```python
from build123d import *

# Parameters (mm, degrees)
SKETCH1_R          = 8
EXTRUDE1_DEPTH     = 40
SKETCH2_W          = 5
SKETCH2_H          = 3.872152866
CUT_EXTRUDE1_DEPTH = 25
FILLET1_R          = 2.5
CHAMFER1_SIZE      = 1
SKETCH3_R          = 10
EXTRUDE2_DEPTH     = 15
CHAMFER2_SIZE      = 2
SKETCH4_R          = 12.3
EXTRUDE3_DEPTH     = 12
CHAMFER3_SIZE      = 2
SKETCH5_R          = 12.5
EXTRUDE4_DEPTH     = 13
SKETCH6_R          = 14.5
EXTRUDE5_DEPTH     = 20
SKETCH10_W         = 5
SKETCH10_H         = 6.103543743
CUT_EXTRUDE2_DEPTH = 14.4
FILLET2_R          = 2.5
SKETCH9_R          = 8
EXTRUDE6_DEPTH     = 54
SKETCH11_W         = 4
SKETCH11_H         = 18
CUT_EXTRUDE3_DEPTH = 156.968746869
FILLET3_R          = 2
SKETCH12_R         = 7.975
EXTRUDE7_DEPTH     = 23
CHAMFER4_SIZE      = 1


# Some blends are built 0.0001 mm under size
with BuildPart() as part:
    # Sketch1 → Extrude1 (new body)
    with BuildSketch(Plane.XY):
        Circle(SKETCH1_R)
    extrude(amount=-EXTRUDE1_DEPTH)

    # Sketch2 → Cut-Extrude1 (cut)
    with BuildSketch(Plane.XY):
        with Locations((0, 6.936076433)):
            Rectangle(SKETCH2_W, SKETCH2_H)
    extrude(amount=-CUT_EXTRUDE1_DEPTH, mode=Mode.SUBTRACT)

    # Fillet1
    fillet1_edges = [part.edges().sort_by_distance(p)[0] for p in [
        (2.5, 6.299671038, -25),
        (-2.5, 6.299671038, -25),
    ]]
    fillet(fillet1_edges, radius=FILLET1_R - 0.0001)  # a hair under: the kernel refuses the full size

    # Chamfer1
    chamfer1_edges = [part.edges().sort_by_distance(p)[0] for p in [
        (-4.69041576, -6.480740698, 0),
    ]]
    chamfer(chamfer1_edges, length=CHAMFER1_SIZE)

    # Sketch3 → Extrude2 (add)
    with BuildSketch(Plane(origin=(0, 0, -40), x_dir=(-1, 0, 0), z_dir=(0, 0, -1))):
        Circle(SKETCH3_R)
    extrude(amount=EXTRUDE2_DEPTH)

    # Chamfer2
    chamfer2_edges = [part.edges().sort_by_distance(p)[0] for p in [
        (10, 0, -40),
    ]]
    chamfer(chamfer2_edges, length=CHAMFER2_SIZE - 0.0001)  # a hair under: the kernel refuses the full size

    # Sketch4 → Extrude3 (add)
    with BuildSketch(Plane(origin=(0, 0, -55), x_dir=(-1, 0, 0), z_dir=(0, 0, -1))):
        Circle(SKETCH4_R)
    extrude(amount=EXTRUDE3_DEPTH)

    # Chamfer3
    chamfer3_edges = [part.edges().sort_by_distance(p)[0] for p in [
        (12.3, 0, -55),
    ]]
    chamfer(chamfer3_edges, length=CHAMFER3_SIZE)

    # Sketch5 → Extrude4 (add)
    with BuildSketch(Plane(origin=(0, 0, -67), x_dir=(-1, 0, 0), z_dir=(0, 0, -1))):
        with Locations(Location((0, 0, 0), (0, 0, 180))):
            Circle(SKETCH5_R)
    extrude(amount=EXTRUDE4_DEPTH)

    # Sketch6 → Extrude5 (add)
    with BuildSketch(Plane(origin=(0, 0, -80), x_dir=(-1, 0, 0), z_dir=(0, 0, -1))):
        Circle(SKETCH6_R)
    extrude(amount=EXTRUDE5_DEPTH)

    # Sketch10 → Cut-Extrude2 (cut)
    with BuildSketch(Plane.XY.offset(-55)):
        with Locations((0, 13.551771871)):
            Rectangle(SKETCH10_W, SKETCH10_H)
    extrude(amount=-CUT_EXTRUDE2_DEPTH, mode=Mode.SUBTRACT)

    # Fillet2
    # the kernel refuses this fillet: 2.5 mm, written as the material it adds along each edge
    with BuildSketch(Plane(origin=(2.5, 18.497448714, -69.4), x_dir=(0, 0, 1), z_dir=(0, -1, 0))) as fillet2_piece_1_section:
        with BuildLine():
            CenterArc((FILLET2_R, FILLET2_R), FILLET2_R, 180, 90)
            Line((0, FILLET2_R), (0, 0))
            Line((0, 0), (FILLET2_R, 0))
        make_face()
    fillet2_piece_1 = extrude(amount=14.247448714, mode=Mode.PRIVATE)
    fillet2_piece_1 = fillet2_piece_1 & Plane(origin=(0, 0, -68.840122938), x_dir=(1, 0, 0), z_dir=(0, 0, 1)) * Cylinder(12.5, 39, mode=Mode.PRIVATE)
    fillet2_piece_1 = split(fillet2_piece_1, bisect_by=Plane(origin=(1.944027658, 12.237538555, -67), z_dir=(0, 0, -1)), keep=Keep.TOP, mode=Mode.PRIVATE)
    add(fillet2_piece_1)
    with BuildSketch(Plane(origin=(2.5, 18.497448714, -69.4), x_dir=(0, 0, 1), z_dir=(0, -1, 0))) as fillet2_piece_2_section:
        with BuildLine():
            CenterArc((FILLET2_R, FILLET2_R), FILLET2_R, 180, 90)
            Line((0, FILLET2_R), (0, 0))
            Line((0, 0), (FILLET2_R, 0))
        make_face()
    fillet2_piece_2 = extrude(amount=14.247448714, mode=Mode.PRIVATE)
    fillet2_piece_2 = fillet2_piece_2 & Plane(origin=(0, 0, -66.975002686), x_dir=(-1, 0, 0), z_dir=(0, 0, 1)) * Cylinder(12.3, 39, mode=Mode.PRIVATE)
    add(fillet2_piece_2)
    with BuildSketch(Plane(origin=(-2.5, 4.25, -69.4), x_dir=(1, 0, 0), z_dir=(0, 1, 0))) as fillet2_piece_3_section:
        with BuildLine():
            CenterArc((FILLET2_R, -FILLET2_R), FILLET2_R, 90, 90)
            Line((0, -FILLET2_R), (0, 0))
            Line((0, 0), (FILLET2_R, 0))
        make_face()
    fillet2_piece_3 = extrude(amount=14.247448714, mode=Mode.PRIVATE)
    fillet2_piece_3 = fillet2_piece_3 & Plane(origin=(0, 0, -68.853362748), x_dir=(1, 0, 0), z_dir=(0, 0, 1)) * Cylinder(12.5, 39, mode=Mode.PRIVATE)
    fillet2_piece_3 = split(fillet2_piece_3, bisect_by=Plane(origin=(-1.922744222, 11.319637846, -67), z_dir=(0, 0, -1)), keep=Keep.TOP, mode=Mode.PRIVATE)
    add(fillet2_piece_3)
    with BuildSketch(Plane(origin=(-2.5, 4.25, -69.4), x_dir=(1, 0, 0), z_dir=(0, 1, 0))) as fillet2_piece_4_section:
        with BuildLine():
            CenterArc((FILLET2_R, -FILLET2_R), FILLET2_R, 90, 90)
            Line((0, -FILLET2_R), (0, 0))
            Line((0, 0), (FILLET2_R, 0))
        make_face()
    fillet2_piece_4 = extrude(amount=14.247448714, mode=Mode.PRIVATE)
    fillet2_piece_4 = fillet2_piece_4 & Plane(origin=(0, 0, -66.975002689), x_dir=(-1, 0, 0), z_dir=(0, 0, 1)) * Cylinder(12.3, 39, mode=Mode.PRIVATE)
    add(fillet2_piece_4)

    # Sketch9 → Extrude6 (add)
    with BuildSketch(Plane(origin=(0, 0, -100), x_dir=(-1, 0, 0), z_dir=(0, 0, -1))):
        with Locations(Location((0, 0, 0), (0, 0, 108.209956864))):
            Circle(SKETCH9_R)
    extrude(amount=EXTRUDE6_DEPTH)

    # Sketch11 → Cut-Extrude3 (cut, through all)
    with BuildSketch(Plane(origin=(0, -5.5, 0), x_dir=(-1, 0, 0), z_dir=(0, 1, 0))):
        with Locations((0, -110)):
            Rectangle(SKETCH11_W, SKETCH11_H)
    extrude(amount=-CUT_EXTRUDE3_DEPTH, mode=Mode.SUBTRACT)

    # Fillet3
    fillet3_edges = [part.edges().sort_by_distance(p)[0] for p in [
        (-2, -6.622983346, -119),
        (2, -6.622983346, -119),
        (-2, -6.622983346, -101),
        (2, -6.622983346, -101),
    ]]
    fillet(fillet3_edges, radius=FILLET3_R - 0.0001)  # a hair under: the kernel refuses the full size

    # Sketch12 → Extrude7 (add)
    with BuildSketch(Plane(origin=(0, 0, -154), x_dir=(-1, 0, 0), z_dir=(0, 0, -1))):
        Circle(SKETCH12_R)
    extrude(amount=EXTRUDE7_DEPTH)

    # Chamfer4
    chamfer4_edges = [part.edges().sort_by_distance(p)[0] for p in [
        (7.975, 0, -177),
    ]]
    chamfer(chamfer4_edges, length=CHAMFER4_SIZE)


solid = part.part
```
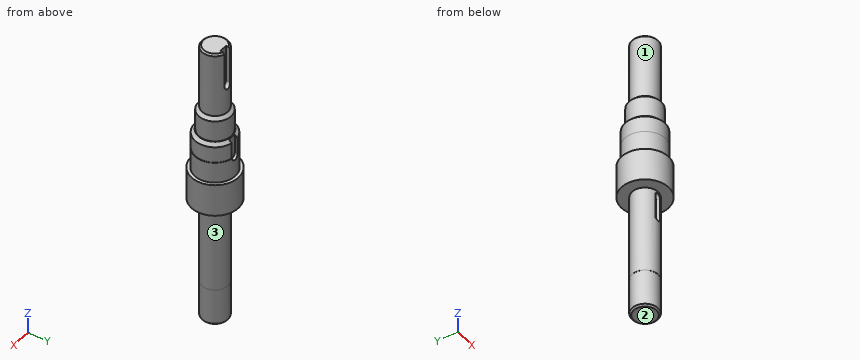
CAD build for the part. Positions are in the model's coordinates, mm. Face numbers are marked on the shaded views. A direction names the side the tool comes from. Coordinates: 2 decimals unless noted, no trailing zeros. Write each loop counter-clockwise with the first axis right and the second up, starting at its lowest first coordinate (ties: lowest second). Pieces come first, ordered by that corner, then holes.
(1) Flat gauge pins, fed straight in: pin 1 (1.8 mm diameter, centred on y = -7, z = -109.5, fed in from -X); pin 2 (2 mm diameter, centred on x = -6.5, z = -93.5, fed in from -Y); pin 3 (10 mm diameter, centred on x = 7, y = 0.5, fed in from -Z); pin 4 (2.5 mm diameter, centred on y = -7, z = -111.5, fed in from +X). Where does each tip first touch, or does it go through?
(2) Cut at C-C, the plane z = -50. List the corners of the cut face in (x, y).
(3) Cut at A-A, the plane z = -83.5. List the corners of the cut face in (x, y), and give its area (3 significant figures).
(4) Cut at B-B, the plane z = -108. List the corners of the cut face in (x, y), and give its area (3 significant figures).
(5) 3-axis set-ups, long thin cutter, end or side, ignore diameter. For the marked faces 1, 2 and 3: which of +Z, -Z, +X, -X, +Y, -Y reach the whole face in a straight line?
(6) Cut at D-D, the plane z = -16. List the corners of the cut face in (x, y).
(7) Drill centre lines: probe 1 along Z at (x, y) = (4.25, 12.5); probe 2 along X at (y, z) = (-2.25, -140); probe 3 along Z at (x, y) = (-8.75, 2). Where is each one in solid material? Low to high.
Geometry says:
1. pin 1: stops at x = -5.18
1. pin 2: stops at y = -13.42
1. pin 3: stops at z = -177
1. pin 4: stops at x = 5.56
2. outline: circle Ø20 at (0, 0)
3. outline: circle Ø29 at (0, 0)
3. area: 661 mm2
4. outline: (-2, -7.75) - (-2, -5.5) - (2, -5.5) - (2, -7.75) arc R8 ccw (long way) to start
4. area: 191 mm2
5. face 1: +Z
5. face 2: -Z, +X, -X, +Y, -Y
5. face 3: -Z
6. outline: (-2.5, 5) - (-2.5, 7.6) arc R8 ccw (long way) to (2.5, 7.6) - (2.5, 5) - close
7. probe 1: z = -100 to -80
7. probe 2: x = -7.68 to 7.68
7. probe 3: z = -100 to -40.98
